from build123d import *

# Parameters (mm, degrees)
SKETCH1_R           = 20.6
BOSS_EXTRUDE1_DEPTH = 2
SKETCH2_R           = 5.15
CUT_EXTRUDE1_DEPTH  = 3
SKETCH3_R           = 6.5
CUT_EXTRUDE2_DEPTH  = 2
BOSS_EXTRUDE4_DEPTH = 22
FILLET1_R           = 5


with BuildPart() as part:
    # Sketch1 → Boss-Extrude1 (new body)
    with BuildSketch(Plane(origin=(0, 0, 0), x_dir=(1, 0, 0), z_dir=(0, 1, 0))):
        with Locations(Location((0, 0, 0), (0, 0, 270))):
            Circle(SKETCH1_R)
    extrude(amount=BOSS_EXTRUDE1_DEPTH)

    # Sketch2 → Cut-Extrude1 (cut)
    with BuildSketch(Plane(origin=(0, 2, 0), x_dir=(1, 0, 0), z_dir=(0, 1, 0))):
        with Locations(Location((0, 0, 0), (0, 0, 270))):
            Circle(SKETCH2_R)
    extrude(amount=-CUT_EXTRUDE1_DEPTH, mode=Mode.SUBTRACT)

    # Sketch3 → Cut-Extrude2 (cut)
    with BuildSketch(Plane(origin=(0, 2, 0), x_dir=(1, 0, 0), z_dir=(0, 1, 0))):
        with Locations(Location((0, 13, 0), (0, 0, 270))):
            Circle(SKETCH3_R)
    extrude(amount=-CUT_EXTRUDE2_DEPTH, mode=Mode.SUBTRACT)

    # Sketch4 → Boss-Extrude4 (add)
    with BuildSketch(Plane(origin=(0, 2, 0), x_dir=(1, 0, 0), z_dir=(0, 1, 0))):
        with BuildLine():
            Line((-16.743954133, 12), (-3.5, 5.5))
            Line((-3.5, 5.5), (3.5, 5.5))
            Line((3.5, 5.5), (16.743954133, 12))
            ThreePointArc((16.743954133, 12), (13.279606143, 15.748398671), (9, 18.529975715))
            ThreePointArc((9, 18.529975715), (0, 6.042759079), (-9, 18.529975715))
            ThreePointArc((-9, 18.529975715), (-13.279606143, 15.748398671), (-16.743954133, 12))
        make_face()
    extrude(amount=BOSS_EXTRUDE4_DEPTH)

    # Fillet1
    # the kernel refuses this fillet: 5 mm, written as the material it takes off along each edge
    with BuildSketch(Plane(origin=(-9, 2, -18.529975715), x_dir=(-0.7582820448894503, 0, 0.6519266372823508), z_dir=(0, 1, 0))) as fillet1_piece_1:
        with BuildLine():
            CenterArc((9.235650387, 4.834535828), FILLET1_R, 166.800937992, 117.98025937)
            ThreePointArc((4.367737182, 5.976210486), (2.790781466, 2.544540557), (0, 0))
            ThreePointArc((0, 0), (5.255646353, -0.681712388), (10.511292706, 0))
        make_face()
    extrude(amount=48.278231764, mode=Mode.SUBTRACT)
    with BuildSketch(Plane(origin=(9, 2, -18.529975715), x_dir=(0.7582820448894505, 0, 0.6519266372823505), z_dir=(0, 1, 0))) as fillet1_piece_2:
        with BuildLine():
            CenterArc((9.235650387, -4.834535828), FILLET1_R, 75.218802639, 117.98025937)
            ThreePointArc((4.367737182, -5.976210486), (2.790781466, -2.544540557), (0, 0))
            ThreePointArc((0, 0), (5.255646353, 0.681712388), (10.511292706, 0))
        make_face()
    extrude(amount=48.278231764, mode=Mode.SUBTRACT)


solid = part.part
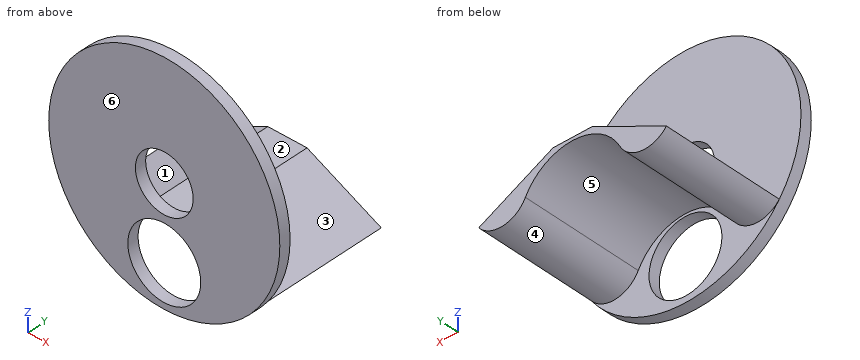
Here's how the part is built. I have some questions about the finished solid (model axes, mm). Face numbers are marked on the shaded views. A direction names the side the tool comes from. Round coordinates to 2 decimals unless told otherwise and drop trailing zeros. Loops run counter-clockwise (first coordinate to the right, second up) from the corner with the lowest first, then second, coordinate; pieces in that order, holes last. Notation, with made-up numbers: M -18.75,-2.5 L 1.25,-2.5 A22 cw 1.25,32.5 Z; hole C 73,17 d2. An arc over 180 degrees is marked long. Write each question's results on one line, items separated by ' | '. Start each with the question number.
(1) I want a section at C-C (y = 15.75). Please give me the cut outline in (x, z), then the cut area to 3 significant figures.
(2) Thinking about a two-plate mould opening in X: for the marked faces 1, 2, 3 and 4, which applies, pulls with the +X half, pulls with the -X half, needs draft (parallel to the pull), parting line crosses it, or undercut?
(3) I want a section at D-D (z = -16). Please give me the cut outline in (x, y), then the cut area to 3 significant figures.
(4) On a 3-axis mill with a long thin cutter (end or side, diameter ignored), from which of +Z, -Z, +X, -X, +Y, -Y can I reach the whole of each face in a straight line? I mean the marked faces 5 and 6. Say none if no direction works.
(5) If I drill on probe 1 along X at (y, z) = (0.5, 0); probe 2 along Y at (x, z) = (-4, 5.5); probe 3 along X at (y, z) = (1.45, -13), over which ranges is the centre line in solid material (lowest first)? Write a range as from..to.
(6) Will these pins go through, and if not, where does the flat tip stop? P1, Ø5, axis at x = 0.5, y = 17, coming from the -Z side; P2, Ø9.5, axis at x = 0, z = 0, coming from the -Y side; P3, Ø2, axis at x = -1, y = 9, coming from the +Z side; P4, Ø12, axis at x = -3, y = 15, coming from the -Z side.
(7) I want a section at A-A (z = 0). Please give me the cut outline in (x, y).
(8) I want a section at B-B (x = 0). Please give me the cut outline in (y, z).
Solved:
1) outline: M -16.73,-11.99 A5 ccw -8.42,-11.15 A9.49 cw 8.42,-11.15 A5 ccw 16.73,-11.99 L 3.5,-5.5 L -3.5,-5.5 Z | area: 75.4 mm²
2) face 1: pulls with the -X half | face 2: needs draft | face 3: pulls with the +X half | face 4: undercut
3) outline: M -12.98,0 L -5.77,0 L -5.77,2 L -12.98,2 Z; M 5.77,0 L 12.98,0 L 12.98,2 L 5.77,2 Z | area: 28.8 mm²
4) face 5: -Z, +Y | face 6: +Z, -Z, +X, -X, -Y
5) probe 1: x = -20.6..-5.15, 5.15..20.6 | probe 2: y = 0..2 | probe 3: x = -15.98..-6.5, 6.5..15.98
6) P1: stops at z = -6.53 | P2: passes through | P3: stops at z = -5.5 | P4: stops at z = -12.03
7) outline: M -20.6,0 L -5.15,0 L -5.15,2 L -20.6,2 Z; M 5.15,0 L 20.6,0 L 20.6,2 L 5.15,2 Z
8) outline: M 0,-20.6 L 2,-20.6 L 2,-19.5 L 0,-19.5 Z; M 0,-6.5 L 2,-6.5 L 2,-6.04 L 24,-6.04 L 24,-5.5 L 2,-5.5 L 2,-5.15 L 0,-5.15 Z; M 0,5.15 L 2,5.15 L 2,20.6 L 0,20.6 Z
